CAD build for the part. Positions are in the model's coordinates, mm. Face numbers are marked on the shaded views. A direction names the side the tool comes from. Coordinates: 2 decimals unless noted, no trailing zeros. Order: outer loops, then holes, each group sorted by start corner. A loop starts at its lowest first (then second) coordinate and runs counter-clockwise, first axis right, second up. Notation, with made-up numbers: M 50,-30 L 62,-30 A17 cw 62,-18 Z; hole C 75,-2 d6. An arc over 180 degrees is marked long. Write item = value, one per line.
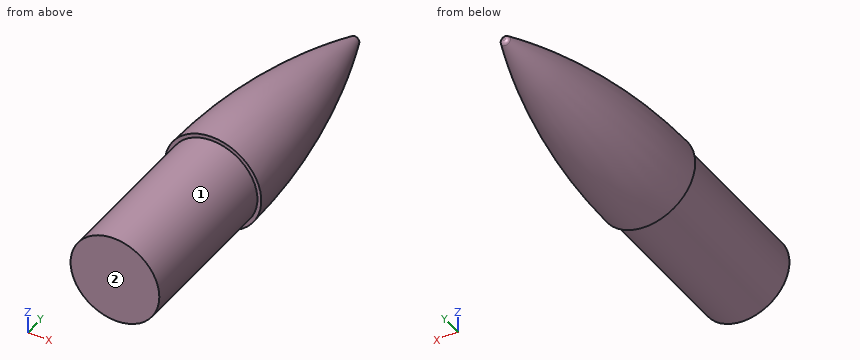
Autodesk Inventor part; units mm, degrees
ref_plane "YZ Plane" through (0, 0, 0) normal (1, 0, 0) x (0, 1, 0)
ref_plane "XZ Plane" through (0, 0, 0) normal (0, 1, 0) x (-1, 0, 0)
ref_plane "XY Plane" through (0, 0, 0) normal (0, 0, 1) x (1, 0, 0)
sketch "Szkic1" plane through (0, 0, 0) normal (0, 0, 1) x (1, 0, 0)
  line L0 (0, 0) -> (-22.98, 0)
  line L1 (-2.0098, 198) -> (0, 198)
  line L2 (0, 198) -> (0, 0)
  line L3 (-22.98, 0) -> (-22.98, 80)
  line L4 (-22.98, 80) -> (-25, 80)
  arc A0 (-2.0098, 198) -> (-25, 80) centre (296.3098, 78.6381) ccw
  dimension "d0" = 22.98
  dimension "d10" = 80
  dimension "d11" = 198
  dimension "d13" = 2.02
revolve "Obrót1" add sketch "Szkic1" angle 360 about axis through (0, 198, 0) along (0, -1, 0)
fillet "Zaokrąglenie2" radius 2 1 edges at (2.0098, 198, 0)
sketch "Szkic4" plane through (0, 0, 0) normal (0, -1, 0) x (1, 0, 0)
  circle A0 centre (0, 0) radius 22.98
  circle A1 centre (0, 0) radius 22.98
  circle A2 centre (0, 0) radius 22.5
  point P0 (0, 0)
  dimension "d21" = 0.48
  dimension "d22" = 45
extrude "parachute" cut sketch "Szkic4" against normal blind 100 contours A2
sketch "Sketch9" plane through (0, 0, 0) normal (0, -1, 0) x (1, 0, 0)
  circle A0 centre (0, 0) radius 22.98
  point P0 (0, 0)
extrude "Extrusion4" add sketch "Sketch9" along normal blind 1
properties part number "nose-conev2" material "Papier"
(1) Wall check: line 1 (Z direction, x = 0, y = 39); line 2 (X direction, y = 64, z = -14); line 3 (X direction, y = 19, z = 8.5). Give the ranges that are in metal, low to high. Write a range as from..to.
Evaluation:
line_1 = -22.98..-22.5, 22.5..22.98
line_2 = -18.22..-17.61, 17.61..18.22
line_3 = -21.35..-20.83, 20.83..21.35
(2) Slice it at A-A, the plane y = 33.5. Write the cut outline in (x, z).
Evaluation:
outline = C 0,0 d45.96; hole C 0,0 d45
(3) Tool access for the marked faces 1 and 2: list every direction of +Z, -Z, +X, -X, +Y, -Y with a clear straight run to the whole face (end or side of a thin tool).
Evaluation:
face_1 = -Y
face_2 = +Z, -Z, +X, -X, -Y
(4) Pin check, flat tips, straight feed: pin 1 Ø4 at (x, y) = (2.5, 67.5) entering from -Z; pin 2 Ø8 at (x, y) = (-7.5, 46.5) entering from +Z; pin 3 Ø2 at (y, z) = (175.5, 5) entering from +X. Stop position of each tip, or through.
Evaluation:
pin_1 = -22.97
pin_2 = 22.71
pin_3 = 9.34
